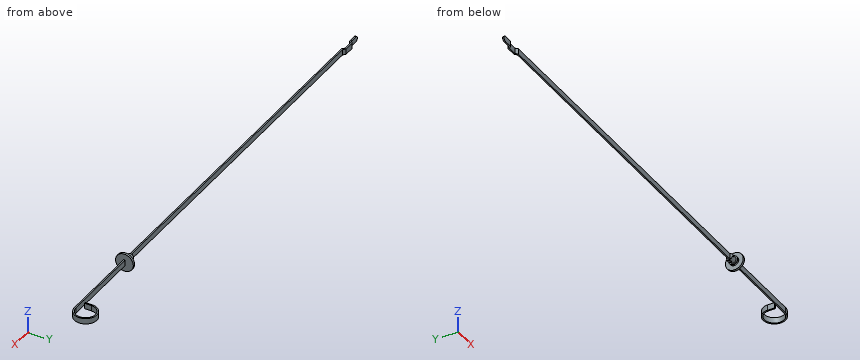
```python
from build123d import *

# Parameters (mm, degrees)
SZKIC6_R                    = 12.7
DODANIE_WYCI_GNI_CIE3_DEPTH = 3
SZKIC7_W                    = 8
SZKIC7_H                    = 2
ZAOKR_GLENIE3_R             = 4
SZKIC13_W                   = 2
SZKIC13_H                   = 5
DODANIE_WYCI_GNI_CIE5_DEPTH = 2
DODANIE_WYCI_GNI_CIE6_START = -5
DODANIE_WYCI_GNI_CIE6_DEPTH = 5


with BuildPart() as part:
    # Szkic5 → Obrót1 (revolve)
    with BuildSketch(Plane.XY):
        with BuildLine():
            Line((0, 6.35), (1, 6.35))
            ThreePointArc((1, 6.35), (2, 5.35), (3, 6.35))
            Line((3, 6.35), (3, 0))
            Line((3, 0), (0, 0))
            Line((0, 0), (-9, 0))
            Line((-9, 0), (-9, 4.35))
            Line((-9, 4.35), (0, 4.35))
            Line((0, 4.35), (0, 6.35))
        make_face()
    revolve(axis=Axis((0, 0, 0), (-1, 0, 0)))

    # Szkic6 → Dodanie-wyciągnięcie3 (add)
    with BuildSketch(Plane(origin=(3, 0, 0), x_dir=(0, 0, -1), z_dir=(1, 0, 0))):
        with Locations(Location((0, 0, 0), (0, 0, 90))):
            Circle(SZKIC6_R)
    extrude(amount=DODANIE_WYCI_GNI_CIE3_DEPTH)

    # Wyciągnięcie po ścieżce1: sweep along a path in Szkic1
    with BuildLine(Plane.XY) as wyci_gni_cie_po_cie_ce1_path:
        Line((110, 5), (110, 15))
        ThreePointArc((110, 15), (135.606601718, 25.606601718), (125, 0))
        Line((125, 0), (0, 0))
        Line((0, 0), (-520, 0))
        Line((-520, 0), (-523, 3))
        Line((-523, 3), (-537, 3))
        Line((-537, 3), (-540, 0))
        Line((-540, 0), (-555, 0))
    # Szkic7 → Wyciągnięcie po ścieżce1 (sweep)
    with BuildSketch(Plane(origin=(0, 0, 0), x_dir=(0, 0, -1), z_dir=(1, 0, 0))):
        Rectangle(SZKIC7_W, SZKIC7_H)
    sweep(path=wyci_gni_cie_po_cie_ce1_path.line, transition=Transition.RIGHT)

    # Zaokrąglenie3
    zaokr_glenie3_edges = [part.edges().sort_by_distance(p)[0] for p in [
        (-555, 0, -4),
        (-555, 0, 4),
    ]]
    fillet(zaokr_glenie3_edges, radius=ZAOKR_GLENIE3_R - 0.0001)  # a hair under: the kernel refuses the full size

    # Szkic13 → Dodanie-wyciągnięcie5 (add)
    with BuildSketch(Plane.ZY.offset(9)):
        with Locations((0, -2.5)):
            Rectangle(SZKIC13_W, SZKIC13_H)
    extrude(amount=-DODANIE_WYCI_GNI_CIE5_DEPTH)

    # Szkic14 → Dodanie-wyciągnięcie6 (add)
    with BuildSketch(Plane.ZY.offset(9).offset(DODANIE_WYCI_GNI_CIE6_START)):
        with BuildLine():
            Line((-2.94595959, 3.200597147), (-4.631919427, 3.814236344))
            Line((-4.631919427, 3.814236344), (-6, 0.055465861))
            Line((-6, 0.055465861), (-4.314040163, -0.558173336))
            ThreePointArc((-4.314040163, -0.558173336), (-4.0876629, 1.487787623), (-2.94595959, 3.200597147))
        make_face()
    extrude(amount=DODANIE_WYCI_GNI_CIE6_DEPTH)


solid = part.part
```
Could you check a few things on this model? Use its own coordinates, in mm. Give positions to 0.01 mm unless a question says otherwise; leave off trailing zeros. Write each loop counter-clockwise with the first axis right and the second up, starting at its lowest first coordinate (ties: lowest second). Pieces come first, ordered by that corner, then holes. Notation, with made-up numbers: (69, 89.5) - (122, 89.5) arc R15 ccw to (122, 115.5) - close; hole circle Ø1 at (-29, 32). An arc over 180 degrees is marked (long way). One line per item, written item: value. Start each with the question number.
Item 1: Imagine slicing it at A-A, the plane y = 23. List the corners of the cut face in (x, z) for me.
Item 2: Please list where these lines run through material, in increasing order: line 1 (Y direction, x = 125, z = 0.25); line 2 (X direction, y = 8, z = -3); line 3 (Z direction, x = 55.5, y = 0). Write a range as from..to.
Item 3: I'm going to push flat-ended pins straight in: pin 1 (12 mm diameter, centred on x = -241.5, z = 0.5, fed in from +Y); pin 2 (10 mm diameter, centred on x = -328, y = 0.5, fed in from +Z); pin 3 (2.5 mm diameter, centred on x = 75, z = -0.5, fed in from -Y); pin 4 (22.5 mm diameter, centred on x = 125, y = 15, fed in from -Z). Where does each tip first touch, or does it pass through?
Item 4: Imagine slicing it at B-B, the plane x = -26.5. List the corners of the cut face in (y, z) for me.
Geometry says:
1. outline: (111.14, -4) - (113.51, -4) - (113.51, 4) - (111.14, 4) - close; (136.49, -4) - (138.86, -4) - (138.86, 4) - (136.49, 4) - close
2. line 1: -1..1, 29..31
2. line 2: 3..6, 109..111, 137.12..139.39
2. line 3: -4..4
3. pin 1: y = 1
3. pin 2: z = 4
3. pin 3: y = -1
3. pin 4: through
4. outline: (-1, -4) - (1, -4) - (1, 4) - (-1, 4) - close
